Can you work these out from the model? Positions are in its coordinate system, mm. Round coordinates to 2 decimals unless told otherwise and drop trailing zeros. Order: outer loops, then holes, each group sorted by start corner. A loop starts at its lowest first (then second) coordinate and runs counter-clockwise, first axis right, second up. Notation, with made-up numbers: M 31,55 L 65,55 A17 ccw 65,60 Z; hole C -4,45.5 d7. An arc over 180 degrees is marked long. Answer as a JSON object with one key per item and string values. Group by question number.
from build123d import *

# Parameters (mm, degrees)
SKETCH1_W           = 50.8
SKETCH1_H           = 50.8
BOSS_EXTRUDE1_DEPTH = 3.175
CUT_EXTRUDE1_DEPTH  = 3.175


with BuildPart() as part:
    # Sketch1 → Boss-Extrude1 (new body)
    with BuildSketch(Plane.XY):
        with Locations((4.943113772, -8.289221557)):
            Rectangle(SKETCH1_W, SKETCH1_H)
    extrude(amount=BOSS_EXTRUDE1_DEPTH)

    # Sketch2 → Cut-Extrude1 (cut)
    with BuildSketch(Plane.XY.offset(3.175)):
        with BuildLine():
            ThreePointArc((19.230613772, -8.289221557), (15.045901909, 1.813566579), (4.943113772, 5.998278443))
            Line((4.943113772, 5.998278443), (4.943113772, -8.289221557))
            Line((4.943113772, -8.289221557), (19.230613772, -8.289221557))
        make_face()
        with BuildLine():
            Line((4.943113772, -8.289221557), (4.943113772, 5.998278443))
            ThreePointArc((4.943113772, 5.998278443), (-5.159674364, 1.813566579), (-9.344386228, -8.289221557))
            Line((-9.344386228, -8.289221557), (4.943113772, -8.289221557))
        make_face()
        with BuildLine():
            Line((19.230613772, -8.289221557), (4.943113772, -8.289221557))
            Line((4.943113772, -8.289221557), (4.943113772, -22.576721557))
            ThreePointArc((4.943113772, -22.576721557), (15.045901909, -18.392009693), (19.230613772, -8.289221557))
        make_face()
        with BuildLine():
            Line((4.943113772, -22.576721557), (4.943113772, -8.289221557))
            Line((4.943113772, -8.289221557), (-9.344386228, -8.289221557))
            ThreePointArc((-9.344386228, -8.289221557), (-5.159674364, -18.392009693), (4.943113772, -22.576721557))
        make_face()
    extrude(amount=-CUT_EXTRUDE1_DEPTH, mode=Mode.SUBTRACT)


solid = part.part
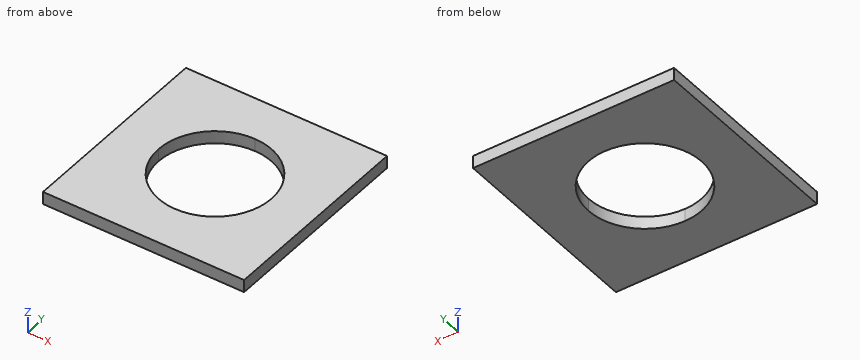
Item 1: Suppose I cut it at A-A, the plane z = 0.9. Write out the boundary of the cut face in (x, y) (1 decimal).
Item 2: Suppose I cut it at C-C, the plane y = -13. Write out the boundary of the cut face in (x, z) (3 decimals), and give its area (3 significant figures).
Item 3: Suppose I cut it at B-B, the plane x = 1.5. Write out the boundary of the cut face in (y, z) (3 decimals), and give its area (3 significant figures).
Item 4: I need wall thicknesses on line 1 (Y direction, x = 4.5, z = 0.8); line 2 (X direction, y = 3, z = 2.8); line 3 (Y direction, x = 14, z = 1.55). Which ranges of each line are inside material? Lowest first, please.
Item 5: I'm going to push a flat-ended pin straight in: pin 1 Ø2 at (x, y) = (5, -21.5) entering from +Z. Where does the tip first touch, or does it pass through?
Computed:
{
 "1": {"outline": "M -20.5,-33.7 L 30.3,-33.7 L 30.3,17.1 L -20.5,17.1 Z; hole C 4.9,-8.3 d28.6"},
 "2": {"outline": "M -20.457,0 L -8.545,0 L -8.545,3.175 L -20.457,3.175 Z; M 18.432,0 L 30.343,0 L 30.343,3.175 L 18.432,3.175 Z", "area": "75.6 mm^2"},
 "3": {"outline": "M -33.689,0 L -22.156,0 L -22.156,3.175 L -33.689,3.175 Z; M 5.577,0 L 17.111,0 L 17.111,3.175 L 5.577,3.175 Z", "area": "73.2 mm^2"},
 "4": {"line 1": "y = -33.69 to -22.57, 5.99 to 17.11", "line 2": "x = -20.46 to -3.81, 13.7 to 30.34", "line 3": "y = -33.69 to -19.34, 2.76 to 17.11"},
 "5": {"pin 1": "passes through"}
}
